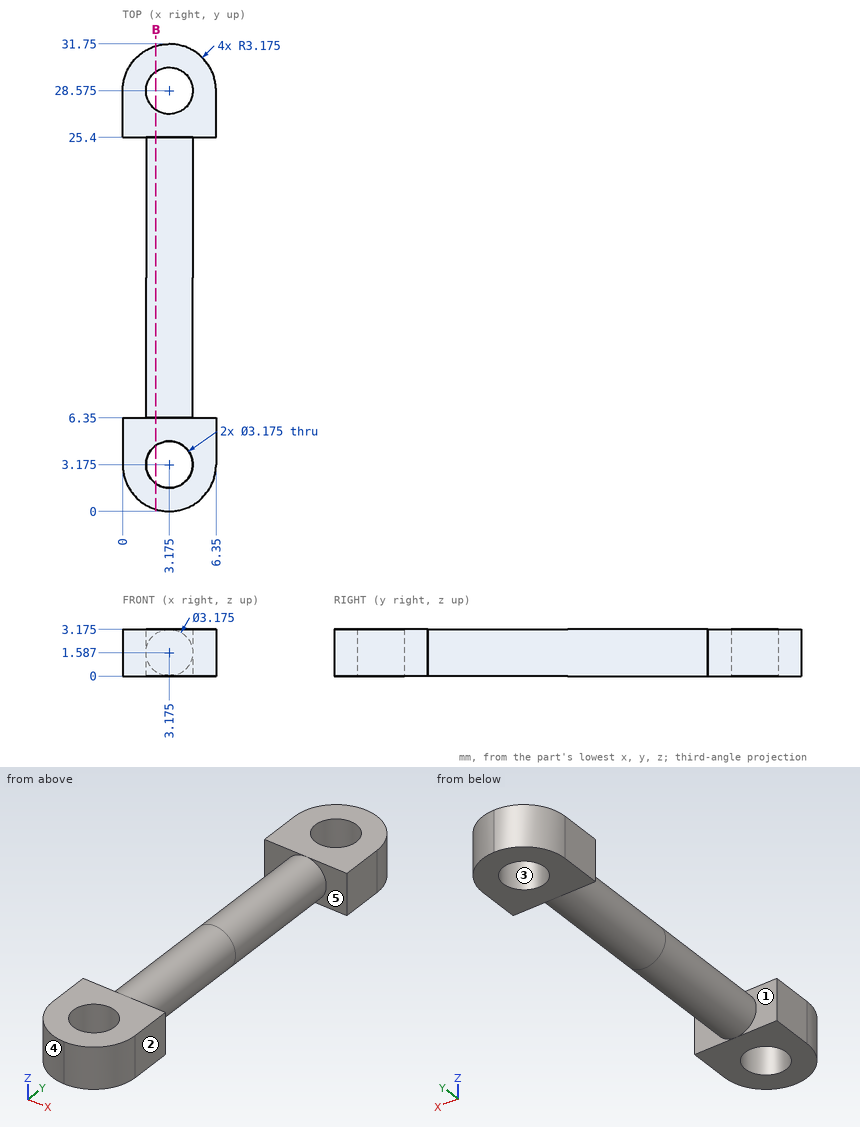
Can you work these out from the drawing? Everything is in mm from the part's minimum corner. A direction names the side the tool comes from. Round coordinates to 2 decimals unless told otherwise and drop trailing zeros. Answer in a Markdown table with one row per item. Add a question column.
(1) I need wall thicknesses on line 1 along Y through (x, z) = (3.5, 2.6); line 2 along Z through (x, y) = (3.25, 23); line 3 along Y through (x, z) = (1, 1.05). Which ranges of each line are inside material? Lowest first, please.
(2) If we section it at B-B (x = 2.25): State how many separate pieces and enclosed holes the cut face has.
(3) For the marked faces 4 and 5, which set-ups out of +Z, -Z, +X, -X, +Y, -Y let a thin tool reach every point of the face, with its end or its side?
(4) If we mould it in two halves opening along X, with no side actions, what happens to the marked faces 1, 2 and 3? For each: pulls with the +X half, pulls with the -X half, needs draft (parallel to the pull), parting line crosses it, or undercut.
(5) I'm going to push a flat-ended pin straight in: pin 1 (1 mm diameter, centred on x = 4.5, z = 1.5, fed in from -Y). Where does the tip first touch, or does it pass through?
Model answer:
| question | item | result |
|---|---|---|
| 1 | line 1 | y = 0.02 to 1.62, 4.73 to 27.02, 30.13 to 31.73 |
| 1 | line 2 | z = 0 to 3.17 |
| 1 | line 3 | y = 0.86 to 6.35, 25.4 to 30.89 |
| 2 | separate pieces | 3 |
| 2 | enclosed holes | 0 |
| 3 | face 4 | +Z, -Z, -X, -Y |
| 3 | face 5 | +X |
| 4 | face 1 | needs draft |
| 4 | face 2 | pulls with the +X half |
| 4 | face 3 | undercut |
| 5 | pin 1 | stops at y = 0.11 |
